from build123d import *

# Parameters (mm, degrees)
SKETCH_R     = 1.5
PAD_DEPTH    = 1.25
CHAMFER_SIZE = 0.2


with BuildPart() as part:
    # Sketch → Pad (new body, symmetric)
    with BuildSketch(Plane.XY):
        Polygon((2.7, -1.558846), (2.7, 1.558846), (0, 3.117691), (-2.7, 1.558846), (-2.7, -1.558846), (0, -3.117691), align=None)
        Circle(SKETCH_R, mode=Mode.SUBTRACT)
    extrude(amount=PAD_DEPTH, both=True)

    # Sketch001 → Groove (revolve, cut)
    with BuildSketch(Plane.YZ):
        Polygon((-2.7, 1.25), (-3.5, 0.78812), (-3.5, 1.25), align=None)
        Polygon((-2.7, -1.25), (-3.5, -0.78812), (-3.5, -1.25), align=None)
    revolve(axis=Axis((0, 0, 0), (0, 0, 1)), mode=Mode.SUBTRACT)

    # Chamfer
    chamfer_edges = [part.edges().sort_by_distance(p)[0] for p in [
        (-1.5, 0, 1.25),
        (-1.5, 0, -1.25),
    ]]
    chamfer(chamfer_edges, length=CHAMFER_SIZE)


solid = part.part
The listing builds one solid part. Answer for the finished solid, in the listing's coordinates (mm). Give positions to 0.01 mm unless a question says otherwise; leave off trailing zeros. Loops run counter-clockwise (first coordinate to the right, second up) from the corner with the lowest first, then second, coordinate; pieces in that order, holes last.
Item 1: A cutting plane is placed at A-A (z = -0.35). Give the vertices of the cut face in (x, y), then the cut area to 3 significant figures.
Derived:
outline: (-2.7, -1.56) - (0, -3.12) - (2.7, -1.56) - (2.7, 1.56) - (0, 3.12) - (-2.7, 1.56) - close; hole circle Ø3 at (0, 0)
area: 18.2 mm2
Item 2: This flat-tipped pin is pushed along its axis until it touches: pin 1 Ø1.5 at (y, z) = (-2, -0.5) entering from +X. Where does it stop, or does it pass through?
Derived:
pin 1: stops at x = 2.7
Item 3: Find the intervals of material crossed by line 1 along X through (y, z) = (0.5, 0.2); line 2 along Y through (x, z) = (-0.5, -0.95); line 3 along Y through (x, z) = (-0.8, -0.35), in increasing order.
Derived:
line 1: x = -2.7 to -1.41, 1.41 to 2.7
line 2: y = -2.83 to -1.41, 1.41 to 2.83
line 3: y = -2.66 to -1.27, 1.27 to 2.66
Item 4: Determine the mould class of faces 1 (the cylindrical face through (-1.5, 0.07, -0.01)), 2 (the flat face through (0, -2, 1.25)), 3 (the conical face through (-2.47, -1.418, -1.165)) for opening direction Y: +Y half, -Y half, draft (parallel to the pull), parting line (faces both ways), or undercut.
Derived:
face 1: undercut
face 2: draft
face 3: -Y half
